Work out the finished part from the listing and answer in its coordinate system (mm). A direction names the side the tool comes from. Give positions to 0.01 mm unless a question says otherwise; leave off trailing zeros. Write item = value, one per line. Start each with the question number.
1. The mould has two halves that part along Y. Classify faces 4 (the face through (4.12, -0.96, -4.34)), 5 (the face through (3.912, -5, 7)), 6 (the face through (4.44, 8.36, 2.63)): released by +Y, released by -Y, zero draft, split by the parting line, or undercut.
2. For faces 1 (the face through (4.978, -2, -3)), 2 (the face through (3.283, -4.4, -1.4)), 3 (the face through (1.695, 4.4, -1.4)), determine the directions among +Z, -Z, +X, -X, +Y, -Y from which every point of the face is accessible in a straight line to the end or side of a thin tool.
3. Consider L1, parallel to Z at x = 4.55, y = 0 (1 decimal); L2, parallel to Z at x = 3.4, y = 1.75; L3, parallel to X at y = -1, z = -4.75. Determine where each line is inside the solid, lowest interval first. Write a range as [from, to].
4. Flat-ended cylindrical pins translate along their axes: pin 1 Ø1 at (x, y) = (1, -5) entering from +Z; pin 2 Ø4 at (y, z) = (1, 1) entering from -X. Find the tip coordinate at first contact, or state that the pin passes through.
```python
from build123d import *


with BuildPart() as part:
    # Sketch3 → bearing-revolution (revolve)
    with BuildSketch(Plane.XY):
        with BuildLine():
            Line((0.3048, 3.175), (4.9784, 3.175))
            Line((4.9784, 3.175), (4.9784, 4.445))
            Line((4.9784, 4.445), (3.28295, 4.445))
            Line((3.28295, 4.445), (3.28295, 6.6675))
            Line((3.28295, 6.6675), (4.9784, 6.6675))
            Line((4.9784, 6.6675), (4.9784, 8.763))
            Line((4.9784, 8.763), (3.9116, 8.763))
            Line((3.9116, 8.763), (3.9116, 7.9375))
            Line((3.9116, 7.9375), (0.3048, 7.9375))
            ThreePointArc((0.3048, 7.9375), (0.089273853, 7.848226147), (0, 7.6327))
            Line((0, 7.6327), (0, 6.6675))
            Line((0, 6.6675), (1.69545, 6.6675))
            Line((1.69545, 6.6675), (1.69545, 4.445))
            Line((1.69545, 4.445), (0, 4.445))
            Line((0, 4.445), (0, 3.4798))
            ThreePointArc((0, 3.4798), (0.089273853, 3.264273853), (0.3048, 3.175))
        make_face()
    revolve(axis=Axis((-4.832058368, 0, 0), (1, 0, 0)))


solid = part.part
```
Verdict:
q1.face_4 = undercut
q1.face_5 = zero draft
q1.face_6 = split by the parting line
q2.face_1 = +Z, -Z, +X, +Y, -Y
q2.face_2 = +X
q2.face_3 = -X
q3.L1 = [-8.8, -6.7], [-4.4, -3.2], [3.2, 4.4], [6.7, 8.8]
q3.L2 = [-7.74, -6.43], [-4.09, -2.65], [2.65, 4.09], [6.43, 7.74]
q3.L3 = [1.7, 3.28]
q4.pin_1 = 6.54
q4.pin_2 = 0.01
